Design review of the part built by this model. Coordinates are the model's own, in mm. A direction names the side the tool comes from. Give positions to 0.01 mm unless a question says otherwise; leave off trailing zeros. Write each loop counter-clockwise with the first axis right and the second up, starting at its lowest first coordinate (ties: lowest second). Pieces come first, ordered by that corner, then holes. Notation, with made-up numbers: (17, -30.75) -> (59, -30.75) arc R35 cw to (59, 2.25) -> close; hole circle Ø10 at (34.25, 79). An arc over 180 degrees is marked (long way). Use CSV: the item, a comma, the result in double quotes.
```python
from build123d import *

# Parameters (mm, degrees)
F1_DEPTH = 3
F2_DEPTH = 11.5
F3_DEPTH = 18.5


with BuildPart() as f1:
    # F0 (on Top) → F1 (new body)
    with BuildSketch(Plane.XY):
        with BuildLine():
            Line((0, 5.5), (0, 0))
            Line((0, 0), (5.5, 0))
            ThreePointArc((5.5, 0), (1.6109127035, 1.6109127035), (0, 5.5))
        make_face()
        with BuildLine():
            ThreePointArc((11, 5.5), (9.3890872965, 1.6109127035), (5.5, 0))
            Line((5.5, 0), (45.5, 0))
            ThreePointArc((45.5, 0), (41.6109127035, 1.6109127035), (40, 5.5))
            Line((40, 5.5), (11, 5.5))
        make_face()
        with BuildLine():
            ThreePointArc((0, 5.5), (1.6109127035, 1.6109127035), (5.5, 0))
            ThreePointArc((5.5, 0), (9.3890872965, 1.6109127035), (11, 5.5))
            Line((11, 5.5), (9.5, 5.5))
            ThreePointArc((9.5, 5.5), (5.5, 1.5), (1.5, 5.5))
            Line((1.5, 5.5), (0, 5.5))
        make_face()
        with BuildLine():
            ThreePointArc((5.5, 11), (1.6109127035, 9.3890872965), (0, 5.5))
            Line((0, 5.5), (1.5, 5.5))
            ThreePointArc((1.5, 5.5), (5.5, 9.5), (9.5, 5.5))
            Line((9.5, 5.5), (11, 5.5))
            ThreePointArc((11, 5.5), (9.3890872965, 9.3890872965), (5.5, 11))
        make_face()
        with BuildLine():
            Line((0, 11), (0, 5.5))
            ThreePointArc((0, 5.5), (1.6109127035, 9.3890872965), (5.5, 11))
            Line((5.5, 11), (0, 11))
        make_face()
        with BuildLine():
            ThreePointArc((51, 5.5), (49.3890872965, 1.6109127035), (45.5, 0))
            Line((45.5, 0), (51, 0))
            Line((51, 0), (51, 5.5))
        make_face()
        with BuildLine():
            ThreePointArc((40, 5.5), (41.6109127035, 1.6109127035), (45.5, 0))
            ThreePointArc((45.5, 0), (49.3890872965, 1.6109127035), (51, 5.5))
            Line((51, 5.5), (49.5, 5.5))
            ThreePointArc((49.5, 5.5), (45.5, 1.5), (41.5, 5.5))
            Line((41.5, 5.5), (40, 5.5))
        make_face()
        with BuildLine():
            ThreePointArc((5.5, 11), (9.3890872965, 9.3890872965), (11, 5.5))
            Line((11, 5.5), (40, 5.5))
            ThreePointArc((40, 5.5), (41.6109127035, 9.3890872965), (45.5, 11))
            Line((45.5, 11), (5.5, 11))
        make_face()
        with BuildLine():
            ThreePointArc((45.5, 11), (41.6109127035, 9.3890872965), (40, 5.5))
            Line((40, 5.5), (41.5, 5.5))
            ThreePointArc((41.5, 5.5), (45.5, 9.5), (49.5, 5.5))
            Line((49.5, 5.5), (51, 5.5))
            ThreePointArc((51, 5.5), (49.3890872965, 9.3890872965), (45.5, 11))
        make_face()
        with BuildLine():
            ThreePointArc((45.5, 11), (49.3890872965, 9.3890872965), (51, 5.5))
            Line((51, 5.5), (51, 11))
            Line((51, 11), (45.5, 11))
        make_face()
    extrude(amount=F1_DEPTH)

    # F0 (on Top) → F2 (join)
    with BuildSketch(Plane.XY):
        with BuildLine():
            ThreePointArc((0, 5.5), (1.6109127035, 1.6109127035), (5.5, 0))
            ThreePointArc((5.5, 0), (9.3890872965, 1.6109127035), (11, 5.5))
            Line((11, 5.5), (9.5, 5.5))
            ThreePointArc((9.5, 5.5), (5.5, 1.5), (1.5, 5.5))
            Line((1.5, 5.5), (0, 5.5))
        make_face()
        with BuildLine():
            ThreePointArc((5.5, 11), (1.6109127035, 9.3890872965), (0, 5.5))
            Line((0, 5.5), (1.5, 5.5))
            ThreePointArc((1.5, 5.5), (5.5, 9.5), (9.5, 5.5))
            Line((9.5, 5.5), (11, 5.5))
            ThreePointArc((11, 5.5), (9.3890872965, 9.3890872965), (5.5, 11))
        make_face()
        with BuildLine():
            ThreePointArc((45.5, 11), (41.6109127035, 9.3890872965), (40, 5.5))
            Line((40, 5.5), (41.5, 5.5))
            ThreePointArc((41.5, 5.5), (45.5, 9.5), (49.5, 5.5))
            Line((49.5, 5.5), (51, 5.5))
            ThreePointArc((51, 5.5), (49.3890872965, 9.3890872965), (45.5, 11))
        make_face()
        with BuildLine():
            ThreePointArc((40, 5.5), (41.6109127035, 1.6109127035), (45.5, 0))
            ThreePointArc((45.5, 0), (49.3890872965, 1.6109127035), (51, 5.5))
            Line((51, 5.5), (49.5, 5.5))
            ThreePointArc((49.5, 5.5), (45.5, 1.5), (41.5, 5.5))
            Line((41.5, 5.5), (40, 5.5))
        make_face()
    extrude(amount=F2_DEPTH)

    # F0 (on Top) → F3 (join)
    with BuildSketch(Plane.XY):
        with BuildLine():
            ThreePointArc((49.5, 5.5), (45.5, 9.5), (41.5, 5.5))
            Line((41.5, 5.5), (49.5, 5.5))
        make_face()
        with BuildLine():
            Line((49.5, 5.5), (41.5, 5.5))
            ThreePointArc((41.5, 5.5), (45.5, 1.5), (49.5, 5.5))
        make_face()
        with BuildLine():
            ThreePointArc((9.5, 5.5), (5.5, 9.5), (1.5, 5.5))
            Line((1.5, 5.5), (9.5, 5.5))
        make_face()
        with BuildLine():
            Line((9.5, 5.5), (1.5, 5.5))
            ThreePointArc((1.5, 5.5), (5.5, 1.5), (9.5, 5.5))
        make_face()
    extrude(amount=F3_DEPTH)


solid = f1.part
```
(1) Clearance check with flat-ended pins moving along their axes: pin 1 (5.5 mm diameter, centred on x = 25.5, y = 5, fed in from +Z); pin 2 (1.5 mm diameter, centred on x = 7, z = 5, fed in from +Y). State where each tip first meets the part, or that it passes through.
Established:
pin 1,"stops at z = 3"
pin 2,"stops at y = 10.95"
(2) Tool access review of faces 4 (the face through (50, 1, 3)), 5 (the face through (48.7, 7.9, 15)), 6 (the face through (1, 10, 3)): name each direction out of +Z, -Z, +X, -X, +Y, -Y from which nothing blocks a thin tool from reaching the whole face with its end or side.
Established:
face 4,"+Z, +X, -Y"
face 5,"+Z"
face 6,"+Z, -X, +Y"
(3) Take a section at A-A (z = 10.5). Write out the cut boundary in (x, y).
Established:
outline,"circle Ø11 at (5.5, 5.5); circle Ø11 at (45.5, 5.5)"
(4) Take a section at B-B (y = 4.75). Write out the cut boundary in (x, z).
Established:
outline,"(0, 0) -> (51, 0) -> (51, 3) -> (50.95, 3) -> (50.95, 11.5) -> (49.43, 11.5) -> (49.43, 18.5) -> (41.57, 18.5) -> (41.57, 11.5) -> (40.05, 11.5) -> (40.05, 3) -> (10.95, 3) -> (10.95, 11.5) -> (9.43, 11.5) -> (9.43, 18.5) -> (1.57, 18.5) -> (1.57, 11.5) -> (0.05, 11.5) -> (0.05, 3) -> (0, 3) -> close"
(5) For line 1 along Z through (x, y) = (6, 10.5); line 2 along X through (y, z) = (10.5, 3.75); line 3 along X through (y, z) = (4.25, 8.5), list the stretches that pass through material, from the lowest coordinate up. Write a range as [from, to].
Established:
line 1,"z = [0, 11.5]"
line 2,"x = [3.21, 7.79], [43.21, 47.79]"
line 3,"x = [0.14, 10.86], [40.14, 50.86]"
(6) Take a section at D-D (y = 2). Write out the cut boundary in (x, z).
Established:
outline,"(0, 0) -> (51, 0) -> (51, 3) -> (49.74, 3) -> (49.74, 11.5) -> (47.44, 11.5) -> (47.44, 18.5) -> (43.56, 18.5) -> (43.56, 11.5) -> (41.26, 11.5) -> (41.26, 3) -> (9.74, 3) -> (9.74, 11.5) -> (7.44, 11.5) -> (7.44, 18.5) -> (3.56, 18.5) -> (3.56, 11.5) -> (1.26, 11.5) -> (1.26, 3) -> (0, 3) -> close"
(7) Take a section at C-C (x = 8.5). Write out the cut boundary in (y, z).
Established:
outline,"(0, 0) -> (11, 0) -> (11, 3) -> (10.11, 3) -> (10.11, 11.5) -> (8.15, 11.5) -> (8.15, 18.5) -> (2.85, 18.5) -> (2.85, 11.5) -> (0.89, 11.5) -> (0.89, 3) -> (0, 3) -> close"
(8) Mouldability with a two-part tool opening along X and no side actions: class faces 1 (the face through (0, 6, 1)), 2 (the face through (25, 0, 1)), 3 (the face through (25, 6, 3)) as +X half, -X half, draft (parallel to the pull), parting line (faces both ways), or undercut.
Established:
face 1,"-X half"
face 2,"draft"
face 3,"undercut"
